Verification items for the finished model (mm, model axes). Coordinates: 2 decimals unless noted, no trailing zeros. Loops run counter-clockwise (first coordinate to the right, second up) from the corner with the lowest first, then second, coordinate; pieces in that order, holes last.
Q1. Material ranges on probe 1 along Y at (x, z) = (-95.25, 1.85), recorded low to high.
Q2. Sectioned sample at A-A (y = 95.25). Enter the section's corners in (x, z).
Q3. Sectioned sample at B-B (x = -6.35). Enter the section's corners in (y, z), then the cut area to 3 significant figures.
Q4. Mould release check, pull along Y, two halves, no side actions. Record for faces 1 (the face through (-92.904, 5.377, 1.252)), 2 (the face through (-1.528, 1.449, 1.252)), 3 (the face through (-52, 52, 0)): +Y half, -Y half, draft (parallel to the pull), parting line (faces both ways), or undercut.
```python
from build123d import *

# Parameters (mm, degrees)
BOSS_EXTRUDE1_DEPTH = 2.54
SKETCH4_R           = 2.54
CUT_EXTRUDE2_DEPTH  = 2.54


with BuildPart() as part:
    # Sketch1 → Boss-Extrude1 (new body)
    with BuildSketch(Plane.XY):
        with BuildLine():
            Line((-96.52, 0), (-5.08, 0))
            ThreePointArc((-5.08, 0), (-1.487897552, 1.487897552), (0, 5.08))
            Line((0, 5.08), (0, 96.52))
            ThreePointArc((0, 96.52), (-1.487897552, 100.112102448), (-5.08, 101.6))
            Line((-5.08, 101.6), (-96.52, 101.6))
            ThreePointArc((-96.52, 101.6), (-100.112102448, 100.112102448), (-101.6, 96.52))
            Line((-101.6, 96.52), (-101.6, 5.08))
            ThreePointArc((-101.6, 5.08), (-100.112102448, 1.487897552), (-96.52, 0))
        make_face()
    extrude(amount=BOSS_EXTRUDE1_DEPTH)

    # Sketch4 → Cut-Extrude2 (cut)
    with BuildSketch(Plane.XY):
        with Locations((-95.25, 6.35)):
            Circle(SKETCH4_R)
        with Locations(Location((-6.35, 6.35, 0), (0, 0, 180))):
            Circle(SKETCH4_R)
        with Locations((-6.35, 95.25)):
            Circle(SKETCH4_R)
        with Locations(Location((-95.25, 95.25, 0), (0, 0, 180))):
            Circle(SKETCH4_R)
    extrude(amount=CUT_EXTRUDE2_DEPTH, mode=Mode.SUBTRACT)


solid = part.part
```
Geometry check:
1. probe 1: y = 0 to 3.81, 8.89 to 92.71, 97.79 to 101.6
2. outline: (-101.6, 0) - (-97.79, 0) - (-97.79, 2.54) - (-101.6, 2.54) - close; (-92.71, 0) - (-8.89, 0) - (-8.89, 2.54) - (-92.71, 2.54) - close; (-3.81, 0) - (0, 0) - (0, 2.54) - (-3.81, 2.54) - close
3. outline: (0, 0) - (3.81, 0) - (3.81, 2.54) - (0, 2.54) - close; (8.89, 0) - (92.71, 0) - (92.71, 2.54) - (8.89, 2.54) - close; (97.79, 0) - (101.6, 0) - (101.6, 2.54) - (97.79, 2.54) - close
3. area: 232 mm2
4. face 1: undercut
4. face 2: -Y half
4. face 3: draft
